```python
from build123d import *

# Parameters (mm, degrees)
SKETCH1_R               = 38.1
BOSS_EXTRUDE1_DEPTH     = 25.4
CUT_EXTRUDE1_REACH      = 141.122
CUT_EXTRUDE1_END_RADIUS = 38.1
CUT_EXTRUDE3_DEPTH      = 6.35


with BuildPart() as part:
    # Sketch1 → Boss-Extrude1 (new body)
    with BuildSketch(Plane(origin=(0, 0, 0), x_dir=(1, 0, 0), z_dir=(0, 1, 0))):
        with BuildLine():
            Line((-57.15, 50.8), (57.15, 50.8))
            ThreePointArc((57.15, 50.8), (61.640128061, 48.940128061), (63.5, 44.45))
            Line((63.5, 44.45), (63.5, -44.45))
            ThreePointArc((63.5, -44.45), (61.640128061, -48.940128061), (57.15, -50.8))
            Line((57.15, -50.8), (-57.15, -50.8))
            ThreePointArc((-57.15, -50.8), (-61.640128061, -48.940128061), (-63.5, -44.45))
            Line((-63.5, -44.45), (-63.5, 44.45))
            ThreePointArc((-63.5, 44.45), (-61.640128061, 48.940128061), (-57.15, 50.8))
        make_face()
        with Locations(Location((0, 0, 0), (0, 0, 270))):
            Circle(SKETCH1_R, mode=Mode.SUBTRACT)
    extrude(amount=BOSS_EXTRUDE1_DEPTH)

    # Cut-Extrude1: up to this cylinder (the profile starts outside it)
    cut_extrude1_end = Plane(origin=(0, 12.7, 0), z_dir=(0, -1, 0)) * Cylinder(CUT_EXTRUDE1_END_RADIUS, 359.444, mode=Mode.PRIVATE)
    # Sketch2 → Cut-Extrude1 (cut, up to the surface)
    with BuildSketch(Plane(origin=(63.5, 0, 0), x_dir=(0, 0, -1), z_dir=(1, 0, 0)), mode=Mode.PRIVATE) as cut_extrude1_sk1:
        Polygon((8.146406132, 12.7), (4.073203066, 19.75499466), (-4.073203066, 19.75499466), (-8.146406132, 12.7), (-4.073203066, 5.64500534), (4.073203066, 5.64500534), align=None)
    cut_extrude1_tool1 = extrude(cut_extrude1_sk1.sketch, amount=-CUT_EXTRUDE1_REACH, mode=Mode.PRIVATE) - cut_extrude1_end
    add(cut_extrude1_tool1.solids().sort_by_distance((63.5, 12.7, 0))[0], mode=Mode.SUBTRACT)

    # Sketch3 → Cut-Extrude3 (cut)
    with BuildSketch(Plane(origin=(0, 0, -50.8), x_dir=(-1, 0, 0), z_dir=(0, 0, -1))):
        Polygon((0, 22.327483366), (10.590327972, 3.984497249), (-10.590327972, 3.984497249), align=None)
    extrude(amount=-CUT_EXTRUDE3_DEPTH, mode=Mode.SUBTRACT)


solid = part.part
```
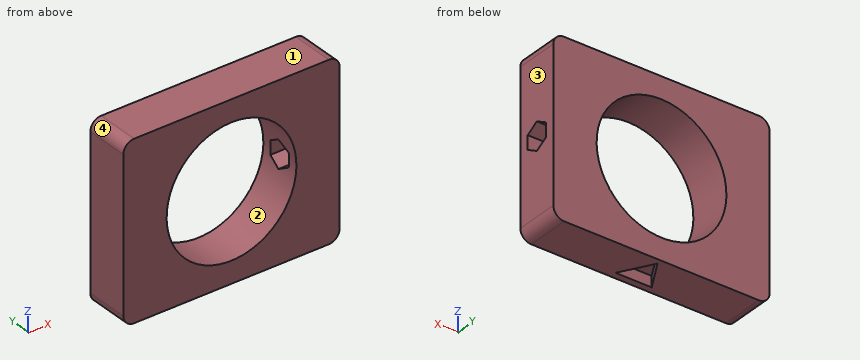
Part model, mm, in its own coordinate system. Face numbers are marked on the shaded views. Round coordinates to 2 decimals unless told otherwise and drop trailing zeros. Order: outer loops, then holes, each group sorted by start corner. A loop starts at its lowest first (then second) coordinate and runs counter-clockwise, first axis right, second up. Notation, with made-up numbers: M 27.5,24.25 L 55.5,24.25 A18 ccw 55.5,50.25 Z; hole C 77,14 d5. An arc over 180 degrees is marked long. Answer in a Markdown table with one row per item. Add a question column.
Q1. Cut at D-D on z = -10.5. Give the cut face in (x, y).
Q2. Pin check, flat tip, straight feed: pin 1 (5.5 mm diameter, centred on x = 1.5, y = 11, fed in from -Z). Stop position of the tip, or through.
Q3. Cut at C-C on x = -17. Give the cut face in (y, z).
Q4. Cut at B-B on x = 51. Give the cut face in (y, z) (3 decimals), and give its area (3 significant figures).
Q5. Cut at A-A on z = 0. Give the cut face in (x, y) (3 decimals), and give its area (3 significant figures).
Q6. Mould opens along X. For the marked faces 1, 2, 3 and 4 say: +X half, -X half, draft (parallel to the pull), parting line (faces both ways), or undercut.
Q7. Wall check: L1, parallel to X at y = 20, z = 0; L2, parallel to Z at x = 33.5, y = 13; L3, parallel to X at y = 9.5, z = -8. Give the ranges that are in metal, low to high. Write a range as from..to.
Established:
| question | item | result |
|---|---|---|
| 1 | outline | M -63.5,0 L -36.62,0 L -36.62,25.4 L -63.5,25.4 Z; M 36.62,0 L 63.5,0 L 63.5,25.4 L 36.62,25.4 Z |
| 2 | pin 1 | stops at z = -44.45 |
| 3 | outline | M 0,-50.8 L 25.4,-50.8 L 25.4,-34.1 L 0,-34.1 Z; M 0,34.1 L 25.4,34.1 L 25.4,50.8 L 0,50.8 Z |
| 4 | outline | M 0,-50.8 L 25.4,-50.8 L 25.4,50.8 L 0,50.8 Z; hole M 5.645,-4.073 L 12.7,-8.146 L 19.755,-4.073 L 19.755,4.073 L 12.7,8.146 L 5.645,4.073 Z |
| 4 | area | 2,410 mm2 |
| 5 | outline | M -63.5,0 L -38.1,0 L -38.1,25.4 L -63.5,25.4 Z; M 38.1,0 L 63.5,0 L 63.5,5.645 L 38.1,5.645 Z; M 38.1,19.755 L 63.5,19.755 L 63.5,25.4 L 38.1,25.4 Z |
| 5 | area | 932 mm2 |
| 6 | face 1 | draft |
| 6 | face 2 | undercut |
| 6 | face 3 | +X half |
| 6 | face 4 | -X half |
| 7 | L1 | x = -63.5..-38.1, 38.1..63.5 |
| 7 | L2 | z = -50.8..-18.15, 18.15..50.8 |
| 7 | L3 | x = -63.5..-37.25, 37.25..63.5 |
